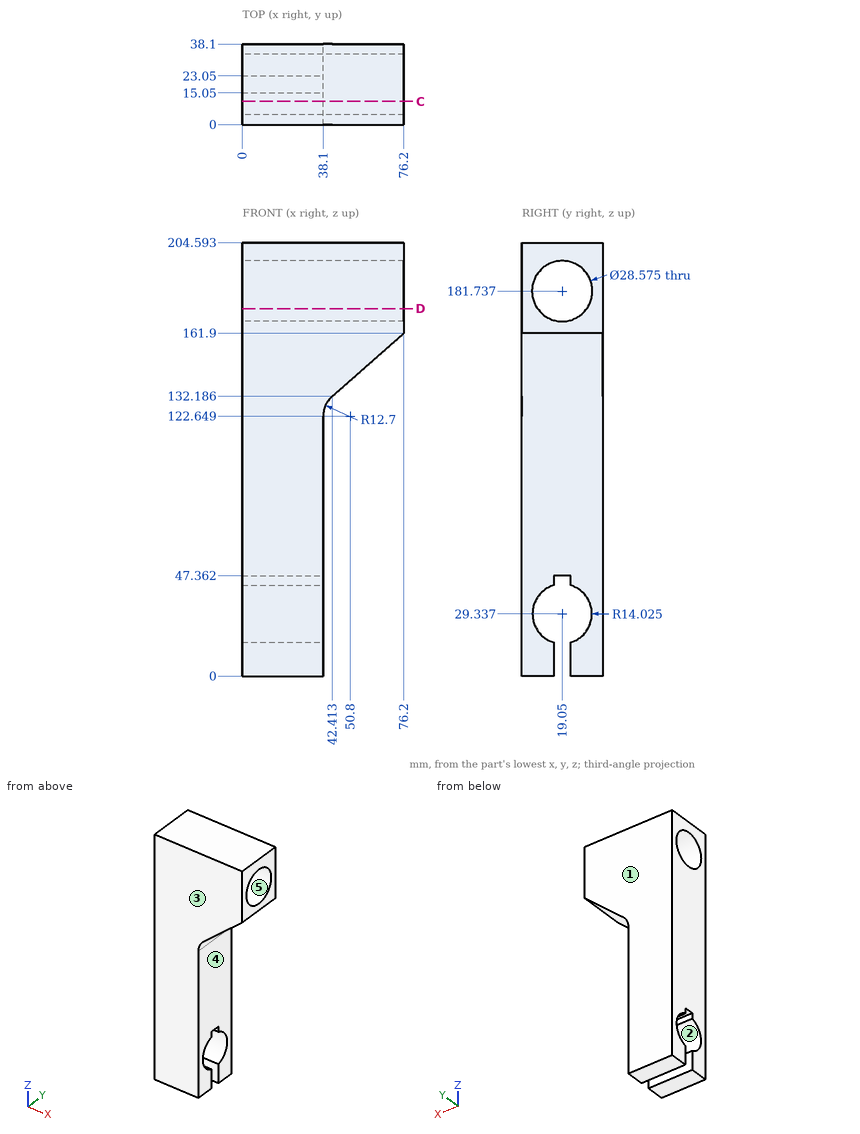
Job drawing, mm, ordinate dimensions from the low corner. One solid piece. A direction names the side the tool comes from. Round coordinates to 2 decimals unless told otherwise and drop trailing zeros. Order: outer loops, then holes, each group sorted by start corner. A loop starts at its lowest first (then second) coordinate and runs counter-clockwise, first axis right, second up. Notation, with made-up numbers: M 89.25,53.25 L 139.25,53.25 A9 cw 139.25,58.25 Z; hole C -33,38 d5. An arc over 180 degrees is marked long. Write each question's results on one line, items separated by ' | '. Start each with the question number.
(1) Two-plate mould, pull along Y, no slides. Class the marked faces 3, 4 and 5: pulls with the +Y half, pulls with the -Y half, needs draft (parallel to the pull), parting line crosses it, or undercut.
(2) Which spindle directions (+Z, -Z, +X, -X, +Y, -Y) get a long thin tool onto all of the face, cutting with end or side? Do the marked faces 1 and 2. Say none if no direction does.
(3) Drop flat-ended pins along their axis: pin 1 (10 mm diameter, centred on y = 24, z = 156.5, fed in from +X) (1 decimal); pin 2 (11.5 mm diameter, centred on y = 26.5, z = 50.5, fed in from +X); pin 3 (8 mm diameter, centred on x = 46.5, y = 15.5, fed in from -Z). Give the stop position or say it passes through.
(4) Probe probe 1 along Z at (x, y) = (18.5, 6.5) (1 decimal); probe 2 along Z at (x, y) = (27.5, 11) (1 decimal); probe 3 along Y at (x, z) = (7.5, 27). List the from-to ranges inside material, lowest first. Write a range as from..to.
(5) Saw through at C-C, the plane y = 11. Give the cut face in (x, z), then the cut area to 3 significant figures.
(6) Saw through at D-D, the plane z = 173.5. Give the cut face in (x, y).
Established:
1) face 3: pulls with the -Y half | face 4: needs draft | face 5: undercut
2) face 1: +Z, -Z, +X, -X, +Y | face 2: +X, -X
3) pin 1: stops at x = 75.7 | pin 2: stops at x = 38.1 | pin 3: stops at z = 132.26
4) probe 1: z = 0..23.1, 35.6..174.9, 188.6..204.6 | probe 2: z = 0..17.9, 40.8..169.9, 193.5..204.6 | probe 3: y = 0..5.22, 32.88..38.1
5) outline: M 0,0 L 38.1,0 L 38.1,17.85 L 0,17.85 Z; M 0,40.82 L 38.1,40.82 L 38.1,122.65 A12.7 cw 42.41,132.19 L 76.2,161.9 L 76.2,169.93 L 0,169.93 Z; M 0,193.54 L 76.2,193.54 L 76.2,204.59 L 0,204.59 Z | area: 7,390 mm^2
6) outline: M 0,0 L 76.2,0 L 76.2,7.38 L 0,7.38 Z; M 0,30.72 L 76.2,30.72 L 76.2,38.1 L 0,38.1 Z
